```python
from build123d import *

# Parameters (mm, degrees)
SKETCH1_R           = 3.175
SKETCH1_R_2         = 4.7371
BOSS_EXTRUDE1_DEPTH = 6.35
SKETCH2_W           = 25.498289586
SKETCH2_H           = 6.35
CUT_EXTRUDE1_DEPTH  = 6.35
SKETCH4_R           = 0.635
CUT_EXTRUDE3_DEPTH  = 6.35
SKETCH6_R           = 0.635
CUT_EXTRUDE4_DEPTH  = 6.35


with BuildPart() as part:
    # Sketch1 → Boss-Extrude1 (new body)
    with BuildSketch(Plane.XY):
        Polygon((0, 0), (40.64, 0), (40.64, 63.5), (111.76, 63.5), (111.76, 0), (152.4, 0), (152.4, 69.85), (152.4, 120.65), (111.76, 120.65), (40.64, 120.65), (0, 120.65), (0, 69.85), align=None)
        with Locations((20.32, 95.25)):
            Circle(SKETCH1_R, mode=Mode.SUBTRACT)
        with Locations((67.945, 95.25)):
            Circle(SKETCH1_R_2, mode=Mode.SUBTRACT)
        with Locations((132.08, 19.05)):
            Circle(SKETCH1_R, mode=Mode.SUBTRACT)
        with Locations((20.32, 76.2)):
            Circle(SKETCH1_R, mode=Mode.SUBTRACT)
        with Locations((20.32, 52.3875)):
            Circle(SKETCH1_R, mode=Mode.SUBTRACT)
        with Locations((20.32, 19.05)):
            Circle(SKETCH1_R, mode=Mode.SUBTRACT)
        with Locations((44.1325, 95.25)):
            Circle(SKETCH1_R, mode=Mode.SUBTRACT)
    extrude(amount=BOSS_EXTRUDE1_DEPTH)

    # Sketch2 → Cut-Extrude1 (cut)
    with BuildSketch(Plane.XY.offset(6.35)):
        with Locations((53.389144793, 66.675)):
            Rectangle(SKETCH2_W, SKETCH2_H)
        with Locations((99.010855207, 66.675)):
            Rectangle(SKETCH2_W, SKETCH2_H)
    extrude(amount=-CUT_EXTRUDE1_DEPTH, mode=Mode.SUBTRACT)

    # Sketch4 → Cut-Extrude3 (cut)
    with BuildSketch(Plane.XY.offset(6.35)):
        with Locations((76.2, 66.675)):
            Circle(SKETCH4_R)
    extrude(amount=-CUT_EXTRUDE3_DEPTH, mode=Mode.SUBTRACT)

    # Sketch6 → Cut-Extrude4 (cut)
    with BuildSketch(Plane.XY.offset(6.35)):
        with Locations((10.16, 66.675)):
            Circle(SKETCH6_R)
        with Locations((30.435806054, 66.675)):
            Circle(SKETCH6_R)
        with Locations((121.92, 66.675)):
            Circle(SKETCH6_R)
        with Locations((142.24, 66.675)):
            Circle(SKETCH6_R)
    extrude(amount=-CUT_EXTRUDE4_DEPTH, mode=Mode.SUBTRACT)


solid = part.part
```
Input: part model. Units: mm. Frame: model coordinates. A direction names the side the tool comes from. Give positions to 0.01 mm unless a question says otherwise; leave off trailing zeros. Order: outer loops, then holes, each group sorted by start corner. A loop starts at its lowest first (then second) coordinate and runs counter-clockwise, first axis right, second up.
1. Section C-C on y = 61.5. Return the cut outline in (x, z), and give its area (3 significant figures).
Derived:
outline: (0, 0) - (40.64, 0) - (40.64, 6.35) - (0, 6.35) - close; (111.76, 0) - (152.4, 0) - (152.4, 6.35) - (111.76, 6.35) - close
area: 516 mm2
2. Material intervals for L1, parallel to X at y = 96, z = 2.5; L2, parallel to X at y = 95, z = 5.5; L3, parallel to X at y = 6.5, z = 4, sorted ascending.
Derived:
L1: x = 0 to 17.23, 23.41 to 41.05, 47.22 to 63.27, 72.62 to 152.4
L2: x = 0 to 17.15, 23.49 to 40.97, 47.3 to 63.21, 72.68 to 152.4
L3: x = 0 to 40.64, 111.76 to 152.4
3. Section B-B on x = 20.32. Give the number of separate pieces and of enclosed holes in the cut face, and give its area (3 significant figures).
Derived:
separate pieces: 5
enclosed holes: 0
area: 605 mm2
4. Reachability of faces 4 (the flat face through (76, 63.5, 3)), 5 (the cylindrical face through (19.91, 98.4, 3.13)) from +Z, -Z, +X, -X, +Y, -Y: full face, straight path, thin tool, end or side. Return the list, or none.
Derived:
face 4: +Z, -Z, -Y
face 5: +Z, -Z
5. Mould query, pull axis X, two halves, no side actions, for faces 1 (the flat face through (152.4, 59, 3)), 2 (the flat face through (20, 0, 3)), 3 (the flat face through (66.138, 67, 3)). Classes: released by +X, released by -X, zero draft, split by the parting line, or undercut.
Derived:
face 1: released by +X
face 2: zero draft
face 3: undercut
6. Section A-A on y = 19.05. Return the cut outline in (x, z) (3 decimals).
Derived:
outline: (0, 0) - (17.145, 0) - (17.145, 6.35) - (0, 6.35) - close; (23.495, 0) - (40.64, 0) - (40.64, 6.35) - (23.495, 6.35) - close; (111.76, 0) - (128.905, 0) - (128.905, 6.35) - (111.76, 6.35) - close; (135.255, 0) - (152.4, 0) - (152.4, 6.35) - (135.255, 6.35) - close
7. Pin query (flat end, axial travel): pin 1 (3 mm diameter, centred on x = 94.5, z = 2, fed in from -Y); pin 2 (0.8 mm diameter, centred on x = 121.92, y = 66.675, fed in from -Z); pin 3 (1.9 mm diameter, centred on x = 72.5, z = 3.5, fed in from -Y). Return the tip coordinate at first contact, or that it passes through.
Derived:
pin 1: stops at y = 69.85
pin 2: passes through
pin 3: stops at y = 63.5
